Here's how the part is built. I have some questions about the finished solid (model axes, mm). A direction names the side the tool comes from. Round coordinates to 2 decimals unless told otherwise and drop trailing zeros. Order: outer loops, then holes, each group sorted by start corner. A loop starts at its lowest first (then second) coordinate and runs counter-clockwise, first axis right, second up. Notation, with made-up numbers: M -37,13.5 L 0,13.5 A21 ccw 0,42.5 Z; hole C 76,20 d6. An arc over 180 degrees is marked long. Write item = value, one per line. Start each with the question number.
Item 1: I want a section at D-D, the plane y = 16. List the corners of the cut face in (x, z) for me, plus the area to 3 significant figures.
Item 2: I'm going to push flat-ended pins straight in: P1, Ø1, axis at x = -9.5, z = 0, coming from the -Y side; P2, Ø0.9, axis at x = -5.5, z = -0.5, coming from the +Y side; P3, Ø1.5, axis at x = 6.5, z = 0, coming from the -Y side. Where does each tip first touch, or does it pass through?
Item 3: I want a section at A-A, the plane y = 6.55. List the corners of the cut face in (x, z) for me, plus the area to 3 significant figures.
Item 4: Please list where these lines run through material, in increasing order: L1, parallel to X at y = 15, z = 1.35; L2, parallel to X at y = -15, z = 0.4; L3, parallel to Y at x = 2.5, z = -0.7.
Item 5: I want a section at B-B, the plane z = -0.8. List the corners of the cut face in (x, y) for me.
Item 6: We'd pull the mould along X, two halves only. Please class faces 3 (the face through (-13.29, -8.66, 0.02)), 4 (the face through (6, 7, 1.5)), 5 (the face through (-8, -1.55, 0)): pulls with the +X half, pulls with the -X half, needs draft (parallel to the pull), parting line crosses it, or undercut.
Item 7: For faces 1 (the face through (1.55, -8, 0)), 2 (the face through (6, 7, -1.5)), which set-ups out of +Z, -Z, +X, -X, +Y, -Y let a thin tool reach every point of the face, with its end or its side?
```python
from build123d import *

# Parameters (mm, degrees)
SKETCH1_R           = 25
BOSS_EXTRUDE1_DEPTH = 1.5


with BuildPart() as part:
    # Sketch1 → Boss-Extrude1 (new body, symmetric)
    with BuildSketch(Plane.XY):
        with Locations((6.55, 6.55)):
            Circle(SKETCH1_R)
        Polygon((1.55, 1.55), (15.05, 1.55), (15.05, -1.55), (1.55, -1.55), (1.55, -15.05), (-1.55, -15.05), (-1.55, -1.55), (-15.05, -1.55), (-15.05, 1.55), (-1.55, 1.55), (-1.55, 15.05), (1.55, 15.05), align=None, mode=Mode.SUBTRACT)
    extrude(amount=BOSS_EXTRUDE1_DEPTH, both=True)


solid = part.part
```
Filled in:
q1.outline = M -16.6,-1.5 L 29.7,-1.5 L 29.7,1.5 L -16.6,1.5 Z
q1.area = 139 mm^2
q2.P1 = -13.03
q2.P2 = 28.7
q2.P3 = -18.45
q3.outline = M -18.45,-1.5 L -1.55,-1.5 L -1.55,1.5 L -18.45,1.5 Z; M 1.55,-1.5 L 31.55,-1.5 L 31.55,1.5 L 1.55,1.5 Z
q3.area = 141 mm^2
q4.L1 = -16.98 to -1.55, 1.55 to 30.08
q4.L2 = -6.12 to -1.55, 1.55 to 19.22
q4.L3 = -18.12 to -1.55, 1.55 to 31.22
q5.outline = C 6.55,6.55 d50; hole M -15.05,-1.55 L -1.55,-1.55 L -1.55,-15.05 L 1.55,-15.05 L 1.55,-1.55 L 15.05,-1.55 L 15.05,1.55 L 1.55,1.55 L 1.55,15.05 L -1.55,15.05 L -1.55,1.55 L -15.05,1.55 Z
q6.face_3 = parting line crosses it
q6.face_4 = needs draft
q6.face_5 = undercut
q7.face_1 = +Z, -Z
q7.face_2 = -Z, +X, -X, +Y, -Y
